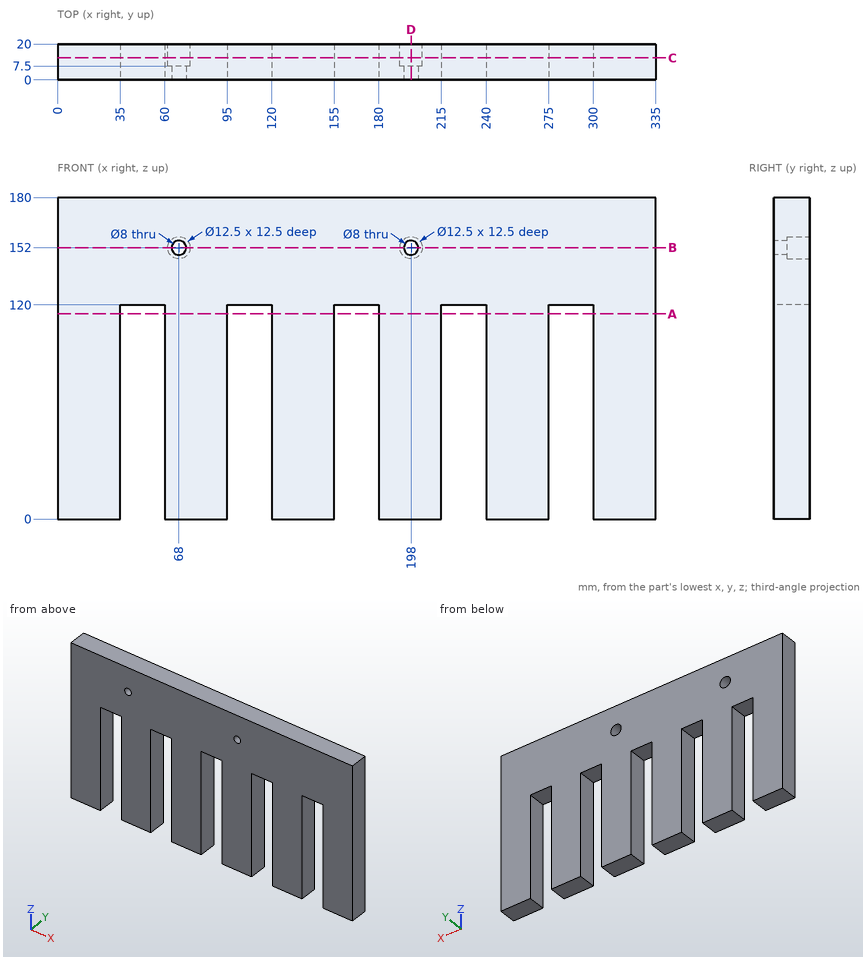
Source: three-view drawing plus pictorial views. Frame: mm from the lowest corner of the part. Coordinates: 2 decimals unless noted, no trailing zeros. Order: outer loops, then holes, each group sorted by start corner. A loop starts at its lowest first (then second) coordinate and runs counter-clockwise, first axis right, second up.
Item 1: Cut plane B-B (z = 152). Return loops of the section in (x, y).
Output values:
outline: (0, 0) - (64, 0) - (64, 7.5) - (61.75, 7.5) - (61.75, 20) - (0, 20) - close; (72, 0) - (194, 0) - (194, 7.5) - (191.75, 7.5) - (191.75, 20) - (74.25, 20) - (74.25, 7.5) - (72, 7.5) - close; (202, 0) - (335, 0) - (335, 20) - (204.25, 20) - (204.25, 7.5) - (202, 7.5) - close
Item 2: Cut plane C-C (y = 12.25). Return loops of the section in (x, z).
Output values:
outline: (0, 0) - (35, 0) - (35, 120) - (60, 120) - (60, 0) - (95, 0) - (95, 120) - (120, 120) - (120, 0) - (155, 0) - (155, 120) - (180, 120) - (180, 0) - (215, 0) - (215, 120) - (240, 120) - (240, 0) - (275, 0) - (275, 120) - (300, 120) - (300, 0) - (335, 0) - (335, 180) - (0, 180) - close; hole circle Ø12.5 at (68, 152); hole circle Ø12.5 at (198, 152)
Item 3: Material intervals for line 1 (X direction, y = 7.75, z = 31); line 2 (X direction, y = 6, z = 152); line 3 (X direction, y = 13.5, z = 152), sorted ascending.
Output values:
line 1: x = 0 to 35, 60 to 95, 120 to 155, 180 to 215, 240 to 275, 300 to 335
line 2: x = 0 to 64, 72 to 194, 202 to 335
line 3: x = 0 to 61.75, 74.25 to 191.75, 204.25 to 335
Item 4: Cut plane A-A (z = 115). Return loops of the section in (x, y), plus the area to 3 significant figures.
Output values:
outline: (0, 0) - (35, 0) - (35, 20) - (0, 20) - close; (60, 0) - (95, 0) - (95, 20) - (60, 20) - close; (120, 0) - (155, 0) - (155, 20) - (120, 20) - close; (180, 0) - (215, 0) - (215, 20) - (180, 20) - close; (240, 0) - (275, 0) - (275, 20) - (240, 20) - close; (300, 0) - (335, 0) - (335, 20) - (300, 20) - close
area: 4,200 mm2
Item 5: Cut plane D-D (x = 198). Return loops of the section in (y, z).
Output values:
outline: (0, 0) - (20, 0) - (20, 145.75) - (7.5, 145.75) - (7.5, 148) - (0, 148) - close; (0, 156) - (7.5, 156) - (7.5, 158.25) - (20, 158.25) - (20, 180) - (0, 180) - close
Item 6: First-contact query: P1, Ø16, axis at x = 68, z = 152, coming from the +Y side; P2, Ø6, axis at x = 283, y = 13.5, coming from the -Z side; P3, Ø9, axis at x = 198, z = 152, coming from the +Y side. Flat tips, straight axial feed; report the tip coordinate or a pass-through.
Output values:
P1: stops at y = 20
P2: stops at z = 120
P3: stops at y = 7.5
